The listing builds one solid part. Answer for the finished solid, in the listing's coordinates (mm). Round coordinates to 2 decimals unless told otherwise and drop trailing zeros. Order: outer loops, then holes, each group sorted by start corner. A loop starts at its lowest first (then second) coordinate and runs counter-clockwise, first axis right, second up. Notation, with made-up numbers: (-16, 89) -> (29, 89) arc R20 ccw to (29, 124) -> close; hole circle Ø8 at (-20, 47). An arc over 180 degrees is marked (long way). Answer in a Markdown table with one row per item. Add a question column.
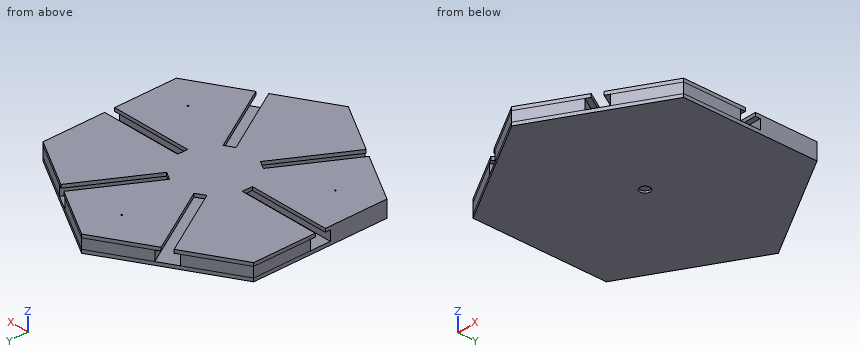
```python
from build123d import *

# Parameters (mm, degrees)
PAD_DEPTH          = 5
PAD001_DEPTH       = 15
PAD003_DEPTH       = 15
POLARPATTERN_COUNT = 6
PAD002_DEPTH       = 5
SKETCH004_R        = 1
POCKET_DEPTH       = 3
SKETCH005_R        = 7.5
POCKET001_DEPTH    = 3


with BuildPart() as part:
    # Sketch → Pad (new body)
    with BuildSketch(Plane.XY):
        Polygon((173.205081, -100), (173.205081, 100), (0, 200), (-173.205081, 100), (-173.205081, -100), (0, -200), align=None)
    extrude(amount=PAD_DEPTH)

    # Sketch001 (on Face8 of Pad) → Pad001 (join)
    with BuildSketch(Plane.XY.offset(5)):
        Polygon((25.980762, -15), (25.980762, 15), (0, 30), (-25.980762, 15), (-25.980762, -15), (0, -30), align=None)
    extrude(amount=PAD001_DEPTH)

    # Sketch003 (on Face5 of Pad001) → Pad003 (join)
    with BuildSketch(Plane.XY.offset(5)):
        Polygon((173.205081, 15), (25.980762, 15), (99.592921, 142.5), (173.205081, 100), align=None)
    pad003 = extrude(amount=PAD003_DEPTH)

    # PolarPattern: Pad003 ×6 about axis
    polarpattern_axis = Axis((0, 0, 5), (0, 0, 1))
    for i in range(1, POLARPATTERN_COUNT):
        add(pad003.rotate(polarpattern_axis, i * 360 / POLARPATTERN_COUNT))

    # Sketch002 (on Face15 of Pad001) → Pad002 (join)
    with BuildSketch(Plane.XY.offset(20)):
        Polygon((0, 200), (80.10735, 153.75), (20.10735, 49.826952), (33.097731, 42.326952), (93.097731, 146.25), (173.205081, 100), (173.205081, 7.5), (53.205081, 7.5), (53.205081, -7.5), (173.205081, -7.5), (173.205081, -100), (93.097731, -146.25), (33.097731, -42.326952), (20.10735, -49.826952), (80.10735, -153.75), (0, -200), (-80.10735, -153.75), (-20.10735, -49.826952), (-33.097731, -42.326952), (-93.097731, -146.25), (-173.205081, -100), (-173.205081, -7.5), (-53.205081, -7.5), (-53.205081, 7.5), (-173.205081, 7.5), (-173.205081, 100), (-93.097731, 146.25), (-33.097731, 42.326952), (-20.10735, 49.826952), (-80.10735, 153.75), align=None)
    extrude(amount=PAD002_DEPTH)

    # Sketch004 (on Face43 of Pad002) → Pocket (cut)
    with BuildSketch(Plane.XY.offset(25)):
        with Locations((0, 140)):
            Circle(SKETCH004_R)
        with Locations((121.243557, -70)):
            Circle(SKETCH004_R)
        with Locations((-121.243557, -70)):
            Circle(SKETCH004_R)
    extrude(amount=-POCKET_DEPTH, mode=Mode.SUBTRACT)

    # Sketch005 (on Face4 of Pocket) → Pocket001 (cut)
    with BuildSketch(Plane(origin=(0, 0, 0), x_dir=(1, 0, 0), z_dir=(0, 0, -1))):
        Circle(SKETCH005_R)
    extrude(amount=-POCKET001_DEPTH, mode=Mode.SUBTRACT)


solid = part.part
```
Item 1: The part is cut by section C-C, the plane x = -134.5. Give the vertices of the cut face in (y, z), and give its area (3 significant figures).
Item 2: The part is cut by section D-D, the plane y = 0. Give the vertices of the cut face in (x, z).
Item 3: Flat-ended cylindrical pins translate along their axes: P1, Ø8, axis at x = 45, z = 17, coming from the -Y side; P2, Ø1, axis at x = -38, z = 17.5, coming from the +Y side; P3, Ø5, axis at y = 0.5, z = 15, coming from the +X side. Find the tip coordinate at first contact, or state that the pin passes through.
Item 4: Find the intervals of material crossed by probe 1 along Y at (x, z) = (-27, 7); probe 2 along Z at (x, y) = (77.5, -109); probe 3 along Y at (x, z) = (33.5, 10), in increasing order. Write a range as [from, to].
Item 5: The part is cut by section B-B, the plane y = 108. Give the vertices of the cut face in (x, z), and give its area (4 significant figures).
Resolved:
| question | item | result |
|---|---|---|
| 1 | outline | (-122.35, 0) -> (122.35, 0) -> (122.35, 25) -> (7.5, 25) -> (7.5, 20) -> (15, 20) -> (15, 5) -> (-15, 5) -> (-15, 20) -> (-7.5, 20) -> (-7.5, 25) -> (-122.35, 25) -> close |
| 1 | area | 5,590 mm2 |
| 2 | outline | (-173.21, 0) -> (-7.5, 0) -> (-7.5, 3) -> (7.5, 3) -> (7.5, 0) -> (173.21, 0) -> (173.21, 5) -> (25.98, 5) -> (25.98, 20) -> (53.21, 20) -> (53.21, 25) -> (-53.21, 25) -> (-53.21, 20) -> (-25.98, 20) -> (-25.98, 5) -> (-173.21, 5) -> close |
| 3 | P1 | y = -176.33 |
| 3 | P2 | y = 178.35 |
| 3 | P3 | x = 25.98 |
| 4 | probe 1 | [-184.41, -76.77], [-16.77, -15], [15, 16.77], [76.77, 184.41] |
| 4 | probe 2 | [0, 5], [20, 25] |
| 4 | probe 3 | [-180.66, -88.02], [-28.02, -15], [15, 28.02], [88.02, 180.66] |
| 5 | outline | (-159.35, 0) -> (159.35, 0) -> (159.35, 25) -> (71.01, 25) -> (71.01, 20) -> (79.67, 20) -> (79.67, 5) -> (45.03, 5) -> (45.03, 20) -> (53.69, 20) -> (53.69, 25) -> (-53.69, 25) -> (-53.69, 20) -> (-45.03, 20) -> (-45.03, 5) -> (-79.67, 5) -> (-79.67, 20) -> (-71.01, 20) -> (-71.01, 25) -> (-159.35, 25) -> close |
| 5 | area | 6,755 mm2 |
